Study the drawing (mm; zero at the part's minimum x, y, z) and answer. A direction names the side the tool comes from. Round coordinates to 2 decimals unless told otherwise and drop trailing zeros. Order: outer loops, then holes, each group sorted by start corner. A loop starts at its lowest first (then second) coordinate and runs counter-clockwise, first axis right, second up. Notation, with made-up numbers: (56, -14) -> (68, -14) arc R19 cw to (68, 23) -> close; hole circle Ø5 at (45, 1.25). An arc over 180 degrees is marked (long way). Answer in a Markdown table with one row per item. Add a question column.
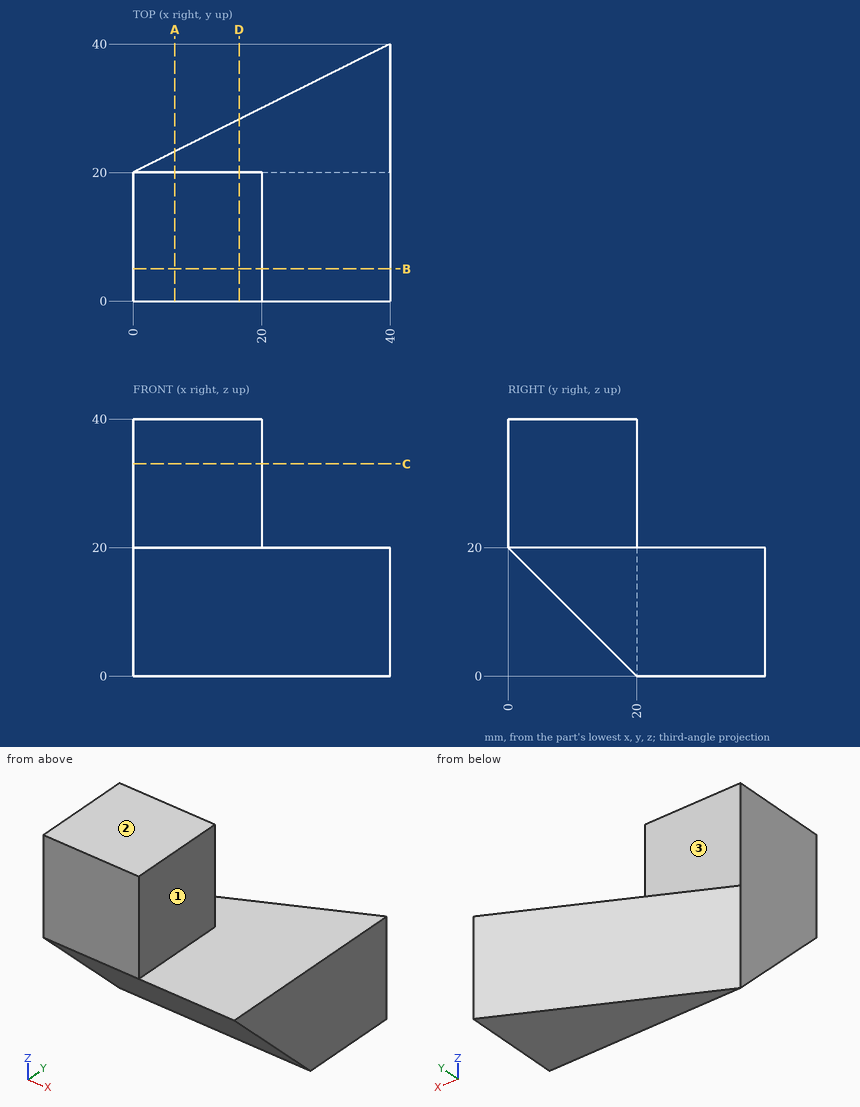
Item 1: The part is cut by section D-D, the plane x = 16.5. Give the vertices of the cut face in (y, z), and give its area (3 significant figures).
Item 2: The part is cut by section A-A, the plane x = 6.5. Give the vertices of the cut face in (y, z), and give its area (3 significant figures).
Item 3: The part is cut by section C-C, the plane z = 33. Give the vertices of the cut face in (x, y), and give its area (3 significant figures).
Item 4: Find the intervals of material crossed by probe 1 along X at (y, z) = (12, 30.5), in increasing order. Write a range as [from, to].
Item 5: The part is cut by section B-B, the plane y = 5. Give the vertices of the cut face in (x, z), and give its area (3 significant figures).
Item 6: Flat-ended cylindrical pins translate along their axes: P1, Ø1.5, axis at x = 17.5, y = 10, coming from the -Z side; P2, Ø12, axis at x = 31, z = 12, coming from the +Y side; P3, Ø1, axis at x = 21, z = 21, coming from the -Y side. Find the tip coordinate at first contact, or state that the pin passes through.
Item 7: A tool of negligible diameter and unlimited length cuts with its end or side. For the marked faces 1, 2 and 3, from which of +Z, -Z, +X, -X, +Y, -Y can it reach the whole face along a straight path? Write none if from no direction.
Resolved:
| question | item | result |
|---|---|---|
| 1 | outline | (0, 20) -> (20, 0) -> (28.25, 0) -> (28.25, 20) -> (20, 20) -> (20, 40) -> (0, 40) -> close |
| 1 | area | 765 mm2 |
| 2 | outline | (0, 20) -> (20, 0) -> (23.25, 0) -> (23.25, 20) -> (20, 20) -> (20, 40) -> (0, 40) -> close |
| 2 | area | 665 mm2 |
| 3 | outline | (0, 0) -> (20, 0) -> (20, 20) -> (0, 20) -> close |
| 3 | area | 400 mm2 |
| 4 | probe 1 | [0, 20] |
| 5 | outline | (0, 15) -> (40, 15) -> (40, 20) -> (20, 20) -> (20, 40) -> (0, 40) -> close |
| 5 | area | 600 mm2 |
| 6 | P1 | z = 9.25 |
| 6 | P2 | y = 38.5 |
| 6 | P3 | through |
| 7 | face 1 | +Z, +X, +Y, -Y |
| 7 | face 2 | +Z, +X, -X, +Y, -Y |
| 7 | face 3 | +Z, +X, -X, +Y |
